Here's how the part is built. I have some questions about the finished solid (model axes, mm). A direction names the side the tool comes from. Round coordinates to 2 decimals unless told otherwise and drop trailing zeros. Order: outer loops, then holes, each group sorted by start corner. A loop starts at its lowest first (then second) coordinate and runs counter-clockwise, first axis right, second up. Notation, with made-up numbers: (54, 38.25) - (82, 38.25) arc R23 cw to (82, 47.25) - close; hole circle Ø7 at (42.5, 31.5). An arc over 180 degrees is marked (long way). Answer as a JSON object with one key per item and string values.
Autodesk Inventor part; units mm, degrees
ref_plane "YZ Plane" through (0, 0, 0) normal (1, 0, 0) x (0, 1, 0)
ref_plane "XZ Plane" through (0, 0, 0) normal (0, 1, 0) x (-1, 0, 0)
ref_plane "XY Plane" through (0, 0, 0) normal (0, 0, 1) x (1, 0, 0)
sketch "Sketch1" plane through (0, 0, 0) normal (0, 1, 0) x (-1, 0, 0)
  line L0 (-70.0685, 0) -> (70.0685, 0) construction
  line L1 (0, -20.6438) -> (0, 20.6438) construction
  line L2 (67.5, -55) -> (-67.5, -55)
  line L3 (-67.5, -55) -> (-67.5, 55)
  line L4 (-67.5, 55) -> (67.5, 55)
  line L5 (67.5, 55) -> (67.5, -55)
  point P0 (0, 0)
  point P1 (0, 0)
  dimension "d0" = 110
  dimension "d1" = 135
extrude "Extrusion1" add sketch "Sketch1" along normal blind 5
sketch "Sketch2" plane through (0, 0, 0) normal (0, -1, 0) x (1, 0, 0)
  line L0 (-161.783, 0) -> (161.783, 0) construction
  line L1 (0, 8.6003) -> (0, -8.6003) construction
  line L2 (-58.2, 45) -> (-54.3, 45) construction
  line L3 (-58.2, 48.05) -> (-54.3, 48.05)
  line L4 (-54.3, 41.95) -> (-58.2, 41.95)
  arc A0 (-58.2, 48.05) -> (-58.2, 41.95) centre (-58.2, 45) ccw
  arc A1 (-54.3, 41.95) -> (-54.3, 48.05) centre (-54.3, 45) ccw
  line L5 (58.2, 45) -> (54.3, 45) construction
  line L6 (58.2, 48.05) -> (54.3, 48.05)
  line L7 (54.3, 41.95) -> (58.2, 41.95)
  arc A2 (58.2, 41.95) -> (58.2, 48.05) centre (58.2, 45) ccw
  arc A3 (54.3, 48.05) -> (54.3, 41.95) centre (54.3, 45) ccw
  line L8 (58.2, -45) -> (54.3, -45) construction
  line L9 (58.2, -41.95) -> (54.3, -41.95)
  line L10 (54.3, -48.05) -> (58.2, -48.05)
  arc A4 (58.2, -48.05) -> (58.2, -41.95) centre (58.2, -45) ccw
  arc A5 (54.3, -41.95) -> (54.3, -48.05) centre (54.3, -45) ccw
  line L11 (-58.2, -45) -> (-54.3, -45) construction
  line L12 (-58.2, -48.05) -> (-54.3, -48.05)
  line L13 (-54.3, -41.95) -> (-58.2, -41.95)
  arc A6 (-58.2, -41.95) -> (-58.2, -48.05) centre (-58.2, -45) ccw
  arc A7 (-54.3, -48.05) -> (-54.3, -41.95) centre (-54.3, -45) ccw
  point P0 (0, 0)
  point P1 (-56.25, 45)
  point P2 (56.25, 45)
  point P3 (56.25, -45)
  point P4 (-56.25, -45)
  point P5 (0, 0)
  point P6 (-61.25, 45)
  point P7 (-51.25, 45)
  dimension "d4" = 112.5
  dimension "d5" = 90
  dimension "d7" = 6.1
  dimension "d8" = 10
extrude "Extrusion2" cut sketch "Sketch2" against normal through all
sketch "Sketch3" plane through (0, 0, 0) normal (0, -1, 0) x (1, 0, 0)
  line L0 (-38.6076, 0) -> (38.6076, 0) construction
  line L1 (0, -3.4177) -> (0, 3.4177) construction
  line L2 (10, -10) -> (-10, -10)
  line L3 (-10, -10) -> (-10, 10)
  line L4 (-10, 10) -> (10, 10)
  line L5 (10, 10) -> (10, -10)
  point P0 (0, 0)
  point P1 (0, 0)
  dimension "d11" = 20
  dimension "d12" = 20
extrude "Extrusion3" add sketch "Sketch3" against normal blind 70
sketch "Sketch4" plane through (-10, 5, 10) normal (0, 0, 1) x (1, 0, 0)
  line L0 (20, 65) -> (0, 65)
  circle A0 centre (10, 65) radius 65
  point P0 (10, -5)
  dimension "d15" = 130
extrude "Extrusion4" add sketch "Sketch4" along normal up to surface (45 mm away)
sketch "Sketch5" plane through (0, 70, 55) normal (0, 0, 1) x (1, 0, 0)
  line L0 (10, 0) -> (-10, 0)
  circle A0 centre (0, 0) radius 35
  point P0 (0, -70)
  dimension "d18" = 70
extrude "Extrusion5" add sketch "Sketch5" along normal blind 35
sketch "Sketch6" plane through (0, 70, 90) normal (0, 0, 1) x (1, 0, 0)
  arc A0 (-2, 6.7082) -> (2, 6.7082) centre (0, 0) ccw
  circle A1 centre (0, 0) radius 35
  line L0 (-2, 8.7082) -> (2, 8.7082)
  line L1 (2, 8.7082) -> (2, 6.7082)
  line L2 (-2, 6.7082) -> (-2, 8.7082)
  point P0 (0, -70)
  dimension "d21" = 14
  dimension "d23" = 2
  dimension "d26" = 4
  dimension "d27" = 2
extrude "Extrusion6" add sketch "Sketch6" along normal blind 30 contours L2 L0 L1 A0
sketch "Sketch8" plane through (-10, 5, 10) normal (0, 0, -1) x (-1, 0, 0)
  arc A0 (-12, 71.7082) -> (-8, 71.7082) centre (-10, 65) ccw
  circle A1 centre (-10, 65) radius 65
  arc A2 (0, 0.7738) -> (-20, 0.7738) centre (-10, 65) ccw
  point P0 (-10, -5)
extrude "Extrusion7" add sketch "Sketch8" along normal blind 135
properties part number "MotorV1"
1. For faces 4 (the face through (28, 42, 55)), 5 (the face through (-1, 2, -55)), 6 (the face through (67.5, 2, -1)), 7 (the face through (-67.5, 2, 1)), 8 (the face through (-61.25, 2.46, 45.07)), which set-ups out of +Z, -Z, +X, -X, +Y, -Y let a thin tool reach every point of the face, with its end or its side?
Responses:
{"face 4": "+Z", "face 5": "-Z, +X, -X, -Y", "face 6": "+Z, -Z, +X, +Y, -Y", "face 7": "+Z, -Z, -X, +Y, -Y", "face 8": "-Y"}
2. For P1, Ø2, axis at x = 55.5, y = 2, coming from the -Z side; P2, Ø12, axis at x = 17.5, y = 31.5, coming from the +Z side; P3, Ø3, axis at y = 109.5, z = -59.5, coming from the -X side, each with a flat end and sliding along its axis, tell me the tip position at first contact or that it passes through.
Responses:
{"P1": "z = -55", "P2": "z = 55", "P3": "x = -52.74"}
3. If I drill on L1, parallel to Z at x = 25, y = 95; L2, parallel to Y at x = -56, z = -36; L3, parallel to Y at x = 9, z = 50, over which ranges is the centre line in solid material (lowest first)? Write a range as [from, to].
Responses:
{"L1": "[-125, 55]", "L2": "[0, 5], [37, 103]", "L3": "[0, 5], [5.63, 134.37]"}
4. Thinking about a two-plate mould opening in Z: for faces 1 (the face through (61.25, 2.46, -45.07)), 2 (the face through (0, 63, 105)), 3 (the face through (1, 2, 55)), which applies, pulls with the +Z half, pulls with the -Z half, needs draft (parallel to the pull), parting line crosses it, or undercut?
Responses:
{"face 1": "undercut", "face 2": "needs draft", "face 3": "pulls with the +Z half"}
5. Imagine slicing it at C-C (y = 96). List the corners of the cut face in (x, z) for me, plus the area to 3 significant figures.
Responses:
{"outline": "(-59.57, -125) - (59.57, -125) - (59.57, 55) - (23.43, 55) - (23.43, 90) - (-23.43, 90) - (-23.43, 55) - (-59.57, 55) - close", "area": "23,100 mm2"}
6. Imagine slicing it at D-D (z = -79). List the corners of the cut face in (x, y) for me, plus the area to 3 significant figures.
Responses:
{"outline": "circle Ø130 at (0, 70)", "area": "13,300 mm2"}
7. Imagine slicing it at B-B (x = 41.5). List the corners of the cut face in (y, z) for me.
Responses:
{"outline": "(0, -55) - (5, -55) - (5, 55) - (0, 55) - close; (19.97, -125) - (120.03, -125) - (120.03, 55) - (19.97, 55) - close"}
8. Imagine slicing it at A-A (z = -45). List the corners of the cut face in (x, y) for me, plus the area to 3 significant figures.
Responses:
{"outline": "(-67.5, 0) - (-61.25, 0) - (-61.25, 5) - (-67.5, 5) - close; circle Ø130 at (0, 70); (-51.25, 0) - (51.25, 0) - (51.25, 5) - (-51.25, 5) - close; (61.25, 0) - (67.5, 0) - (67.5, 5) - (61.25, 5) - close", "area": "13,800 mm2"}
